Part model, mm, in its own coordinate system. Face numbers are marked on the shaded views. A direction names the side the tool comes from. Give positions to 0.01 mm unless a question says otherwise; leave off trailing zeros. Order: outer loops, then holes, each group sorted by start corner. A loop starts at its lowest first (then second) coordinate and runs counter-clockwise, first axis right, second up. Notation, with made-up numbers: (3, 86.25) - (10, 86.25) arc R23 cw to (10, 121.25) - close; hole circle Ø5 at (60, 47). An arc over 180 degrees is marked (long way). One line per item, written item: value.
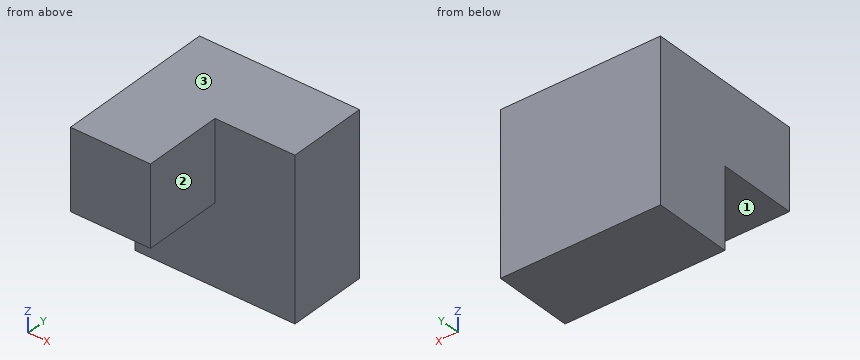
```python
from build123d import *

# Parameters (mm, degrees)
F0_W      = 19.05
F0_H      = 19.05
F1_DEPTH  = 19.05
F2_W      = 38.1
F2_H      = 19.05
F3_DEPTH  = 38.1
F1_FACE_W = 19.05
F1_FACE_H = 19.05
F4_DEPTH  = 19.05
F5_W      = 19.05
F5_H      = 19.05
F6_DEPTH  = 25.4


with BuildPart() as f1:
    # F0 (on Right) → F1 (new body)
    with BuildSketch(Plane.YZ):
        Polygon((-19.05, 0), (0, 0), (0, 38.1), (-19.05, 38.1), (-19.05, 19.05), align=None)
        with Locations((-28.575, 28.575)):
            Rectangle(F0_W, F0_H)
    extrude(amount=-F1_DEPTH)

    # F2 (on Right) → F3 (join)
    with BuildSketch(Plane.YZ):
        with Locations((-19.05, 28.575)):
            Rectangle(F2_W, F2_H)
    extrude(amount=-F3_DEPTH)

    # F1_face (on face) → F4 (join)
    with BuildSketch(Plane(origin=(-19.05, -9.525, 9.525), x_dir=(0, 1, 0), z_dir=(-1, 0, 0))):
        Rectangle(F1_FACE_W, F1_FACE_H)
    extrude(amount=F4_DEPTH)

    # F5 (on face) → F6 (cut)
    with BuildSketch(Plane.XY.offset(38.1)):
        with Locations((-9.525, -28.575)):
            Rectangle(F5_W, F5_H)
    extrude(amount=-F6_DEPTH, mode=Mode.SUBTRACT)


solid = f1.part
```
1) Which spindle directions (+Z, -Z, +X, -X, +Y, -Y) get a long thin tool onto all of the face, cutting with end or side? Do the marked faces 1, 2 and 3. Say none if no direction does.
Outcome:
face 1: -Z, +X, -X, -Y
face 2: +Z, -Z, +X, -Y
face 3: +Z, +X, -X, +Y, -Y
2) Pin check, flat tips, straight feed: pin 1 (12 mm diameter, centred on y = -25.5, z = 13.5, fed in from +X); pin 2 (8 mm diameter, centred on x = -19.5, z = 5.5, fed in from -Y). Stop position of each tip, or through.
Outcome:
pin 1: stops at x = -19.05
pin 2: stops at y = -19.05
3) Drill centre lines: line 1 along Z through (x, y) = (-24.5, -29); line 2 along X through (y, z) = (-23.5, 21.5); line 3 along Y through (x, z) = (-27.5, 16). Where is each one in solid material? Low to high. Write a range as from..to.
Outcome:
line 1: z = 19.05..38.1
line 2: x = -38.1..-19.05
line 3: y = -19.05..0
4) Cut at B-B, the plane y = -25. Give the cut face in (x, z), then the cut area to 3 significant figures.
Outcome:
outline: (-38.1, 19.05) - (-19.05, 19.05) - (-19.05, 38.1) - (-38.1, 38.1) - close
area: 363 mm^2
5) Cut at D-D, the plane z = 33. Give the cut face in (x, y).
Outcome:
outline: (-38.1, -38.1) - (-19.05, -38.1) - (-19.05, -19.05) - (0, -19.05) - (0, 0) - (-38.1, 0) - close
6) Cut at A-A, the plane x = -24. Give the cut face in (y, z).
Outcome:
outline: (-38.1, 19.05) - (-19.05, 19.05) - (-19.05, 0) - (0, 0) - (0, 38.1) - (-38.1, 38.1) - close
7) Cut at C-C, the plane z = 10. Give the cut face in (x, y), then the cut area to 3 significant figures.
Outcome:
outline: (-38.1, -19.05) - (0, -19.05) - (0, 0) - (-38.1, 0) - close
area: 726 mm^2
